Study the drawing (mm; zero at the part's minimum x, y, z) and answer. A direction names the side the tool comes from. Round coordinates to 2 decimals unless told otherwise and drop trailing zeros. Order: outer loops, then holes, each group sorted by start corner. A loop starts at its lowest first (then second) coordinate and runs counter-clockwise, first axis right, second up. Notation, with made-up numbers: M 38.5,28 L 61.5,28 A20 cw 61.5,44 Z; hole C 84.5,67.25 d6. An arc over 180 degrees is marked long. Put each result on its own line as item: value. Start each with the question number.
1. Each of these flat-tipped pins is pushed along its axis until it touches: pin 1 Ø5 at (y, z) = (64, 5.5) entering from +X; pin 2 Ø12 at (y, z) = (25.5, 25) entering from -X; pin 3 Ø4 at (x, y) = (15.5, 21) entering from -Z; pin 4 Ø6 at (x, y) = (4.5, 23.5) entering from +Z. Where does it stop, or does it pass through?
2. The part is cut by section B-B (x = 15). Give the vertices of the cut face in (y, z).
3. The mould has two halves that part along X. Classify the marked faces 4, 5, 6 and 7: +X half, -X half, draft (parallel to the pull), parting line (faces both ways), or undercut.
4. Which of the six approach directions +Z, -Z, +X, -X, +Y, -Y give full straight-line access (tool end or side, diameter ignored) to the marked faces 1, 2 and 3?
5. The part is cut by section A-A (z = 12). Give the vertices of the cut face in (x, y), then the cut area to 3 significant figures.
6. The part is cut by section D-D (z = 15.5). Give the vertices of the cut face in (x, y) (3 decimals).
7. Consider line 1 (Z direction, x = 21, y = 7.5); line 2 (Y direction, x = 15, z = 8.5) (3 decimals); line 3 (Y direction, x = 21.25, z = 26). Determine where each line is inside the solid, lowest interval first.
8. The part is cut by section C-C (y = 24). Give the vertices of the cut face in (x, z), then the cut area to 3 significant figures.
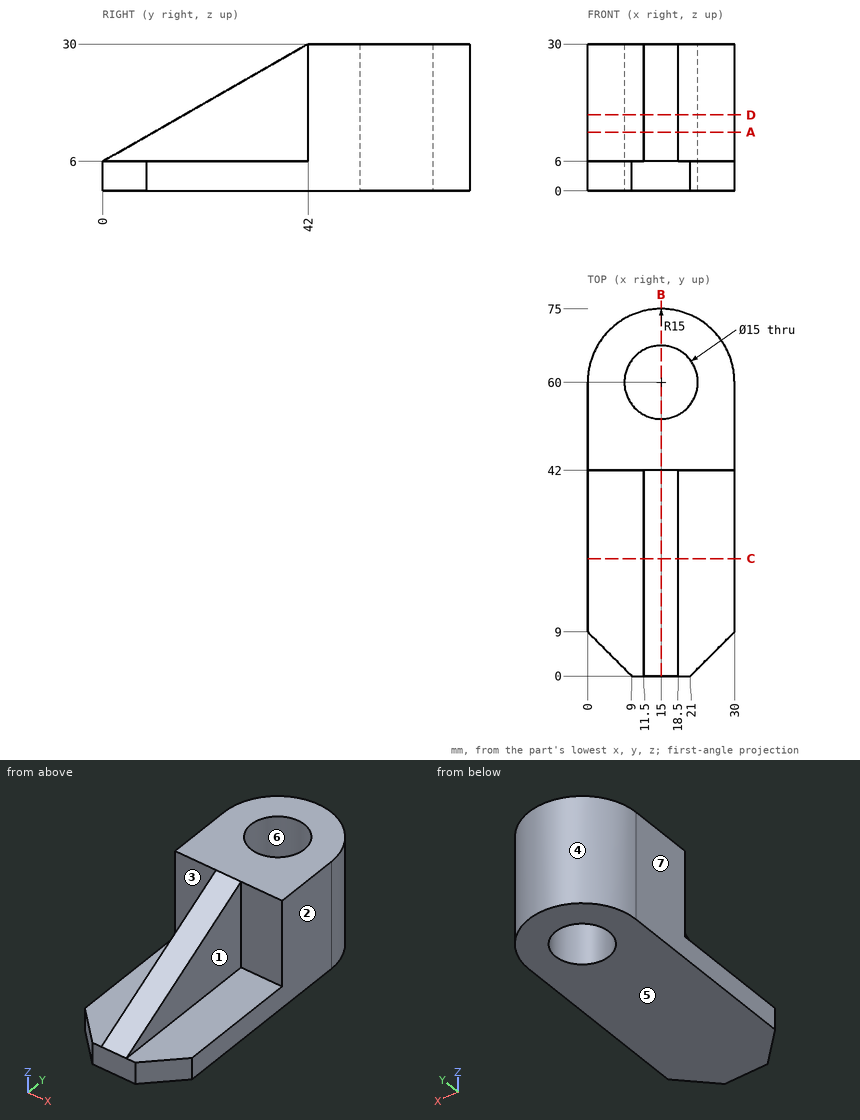
Resolved:
1. pin 1: x = 29.92
1. pin 2: x = 11.5
1. pin 3: z = 0
1. pin 4: z = 6
2. outline: M 0,0 L 52.5,0 L 52.5,30 L 42,30 L 0,6 Z; M 67.5,0 L 75,0 L 75,30 L 67.5,30 Z
3. face 4: parting line
3. face 5: draft
3. face 6: undercut
3. face 7: -X half
4. face 1: +Z, +X, -Y
4. face 2: +Z, -Z, +X, +Y, -Y
4. face 3: +Z, -X, -Y
5. outline: M 0,42 L 11.5,42 L 11.5,10.5 L 18.5,10.5 L 18.5,42 L 30,42 L 30,60 A15 ccw 0,60 Z; hole C 15,60 d15
5. area: 937 mm2
6. outline: M 0,42 L 11.5,42 L 11.5,16.625 L 18.5,16.625 L 18.5,42 L 30,42 L 30,60 A15 ccw 0,60 Z; hole C 15,60 d15
7. line 1: 0 to 6
7. line 2: 4.375 to 52.5, 67.5 to 75
7. line 3: 42 to 55.85, 64.15 to 73.64
8. outline: M 0,0 L 30,0 L 30,6 L 18.5,6 L 18.5,19.71 L 11.5,19.71 L 11.5,6 L 0,6 Z
8. area: 276 mm2
